from build123d import *

# Parameters (mm, degrees)
SKETCH_W     = 104
SKETCH_H     = 33
SKETCH_R     = 1
PAD_DEPTH    = 2
PAD001_DEPTH = 10


with BuildPart() as part:
    # Sketch → Pad (new body)
    with BuildSketch(Plane.XY):
        Rectangle(SKETCH_W, SKETCH_H)
        with Locations((46.9, -11.4)):
            Circle(SKETCH_R, mode=Mode.SUBTRACT)
        with Locations((-46.9, -11.4)):
            Circle(SKETCH_R, mode=Mode.SUBTRACT)
        with Locations((-46.9, 11.4)):
            Circle(SKETCH_R, mode=Mode.SUBTRACT)
        with Locations((46.9, 11.4)):
            Circle(SKETCH_R, mode=Mode.SUBTRACT)
        with BuildLine():
            ThreePointArc((-50, 5.5), (-43.636039, 8.136039), (-41, 14.5))
            Line((41, 14.5), (-41, 14.5))
            ThreePointArc((41, 14.5), (43.636039, 8.136039), (50, 5.5))
            Line((50, -5.5), (50, 5.5))
            ThreePointArc((50, -5.5), (43.636039, -8.136039), (41, -14.5))
            Line((-41, -14.5), (41, -14.5))
            ThreePointArc((-41, -14.5), (-43.636039, -8.136039), (-50, -5.5))
            Line((-50, 5.5), (-50, -5.5))
        make_face(mode=Mode.SUBTRACT)
    extrude(amount=PAD_DEPTH)

    # Sketch → Pad001 (join)
    with BuildSketch(Plane.XY):
        Rectangle(SKETCH_W, SKETCH_H)
        with Locations((46.9, -11.4)):
            Circle(SKETCH_R, mode=Mode.SUBTRACT)
        with Locations((-46.9, -11.4)):
            Circle(SKETCH_R, mode=Mode.SUBTRACT)
        with Locations((-46.9, 11.4)):
            Circle(SKETCH_R, mode=Mode.SUBTRACT)
        with Locations((46.9, 11.4)):
            Circle(SKETCH_R, mode=Mode.SUBTRACT)
        with BuildLine():
            ThreePointArc((-50, 5.5), (-43.636039, 8.136039), (-41, 14.5))
            Line((41, 14.5), (-41, 14.5))
            ThreePointArc((41, 14.5), (43.636039, 8.136039), (50, 5.5))
            Line((50, -5.5), (50, 5.5))
            ThreePointArc((50, -5.5), (43.636039, -8.136039), (41, -14.5))
            Line((-41, -14.5), (41, -14.5))
            ThreePointArc((-41, -14.5), (-43.636039, -8.136039), (-50, -5.5))
            Line((-50, 5.5), (-50, -5.5))
        make_face(mode=Mode.SUBTRACT)
    extrude(amount=PAD001_DEPTH)


solid = part.part
Could you check a few things on this model? Use its own coordinates, in mm. A direction names the side the tool comes from. Coordinates: 2 decimals unless noted, no trailing zeros. Write each loop counter-clockwise with the first axis right and the second up, starting at its lowest first coordinate (ties: lowest second). Pieces come first, ordered by that corner, then holes. Notation, with made-up numbers: (52, 51) - (100, 51) arc R20 cw to (100, 69) - close; hole circle Ø10 at (-30, -0.75). An arc over 180 degrees is marked (long way). Put each result on its own line as item: value. Start each with the question number.
Q1. Thinking about a two-plate mould opening in X: for faces 3 (the flat face through (-1, -16.5, 5)), 4 (the cylindrical face through (43.706, -8.066, 4.93)), 5 (the flat face through (-52, 0, 5)), 6 (the cylindrical face through (-43.706, 8.066, 4.93)), which applies, pulls with the +X half, pulls with the -X half, needs draft (parallel to the pull), parting line crosses it, or undercut?
Q2. I want a section at B-B on y = 4.5. Write out the boundary of the cut face in (x, z), plus the area to 3 significant figures.
Q3. I want a section at A-A on x = 13.5. Write out the boundary of the cut face in (y, z), plus the area to 3 significant figures.
Q4. I'm going to push flat-ended pins straight in: P1, Ø1.6, axis at x = 46.9, y = 11.4, coming from the +Z side; P2, Ø2.5, axis at x = -46.9, y = -11.4, coming from the -Z side. Where does each tip first touch, or does it pass through?
Q5. Which directions (+Z, -Z, +X, -X, +Y, -Y) give clear straight access to the entire face, cutting with the end or side of a thin tool? Please do faces 1 (the flat face through (-1, -14.5, 5)), 2 (the flat face through (-4, -16, 10)).
Q6. I want a section at C-C on z = 8.5. Write out the boundary of the cut face in (x, y).
Q7. Please list where these lines run through material, in increasing order: L1, parallel to Y at x = -40.5, z = 9.25; L2, parallel to X at y = 11.5, z = 3.5; L3, parallel to X at y = 14, z = 5.5.
Q8. I want a section at D-D on y = 11.4. Write out the boundary of the cut face in (x, z).
Checks:
1. face 3: needs draft
1. face 4: undercut
1. face 5: pulls with the -X half
1. face 6: undercut
2. outline: (-52, 0) - (-50, 0) - (-50, 10) - (-52, 10) - close; (50, 0) - (52, 0) - (52, 10) - (50, 10) - close
2. area: 40.0 mm²
3. outline: (-16.5, 0) - (-14.5, 0) - (-14.5, 10) - (-16.5, 10) - close; (14.5, 0) - (16.5, 0) - (16.5, 10) - (14.5, 10) - close
3. area: 40.0 mm²
4. P1: through
4. P2: z = 0
5. face 1: +Z, -Z
5. face 2: +Z, +X, -X, +Y, -Y
6. outline: (-52, -16.5) - (52, -16.5) - (52, 16.5) - (-52, 16.5) - close; hole (-50, -5.5) arc R9 cw to (-41, -14.5) - (41, -14.5) arc R9 cw to (50, -5.5) - (50, 5.5) arc R9 cw to (41, 14.5) - (-41, 14.5) arc R9 cw to (-50, 5.5) - close; hole circle Ø2 at (-46.9, -11.4); hole circle Ø2 at (-46.9, 11.4); hole circle Ø2 at (46.9, -11.4); hole circle Ø2 at (46.9, 11.4)
7. L1: -16.5 to -14.5, 14.5 to 16.5
7. L2: -52 to -47.89, -45.91 to -41.51, 41.51 to 45.91, 47.89 to 52
7. L3: -52 to -41.01, 41.01 to 52
8. outline: (-52, 0) - (-47.9, 0) - (-47.9, 10) - (-52, 10) - close; (-45.9, 0) - (-41.55, 0) - (-41.55, 10) - (-45.9, 10) - close; (41.55, 0) - (45.9, 0) - (45.9, 10) - (41.55, 10) - close; (47.9, 0) - (52, 0) - (52, 10) - (47.9, 10) - close
